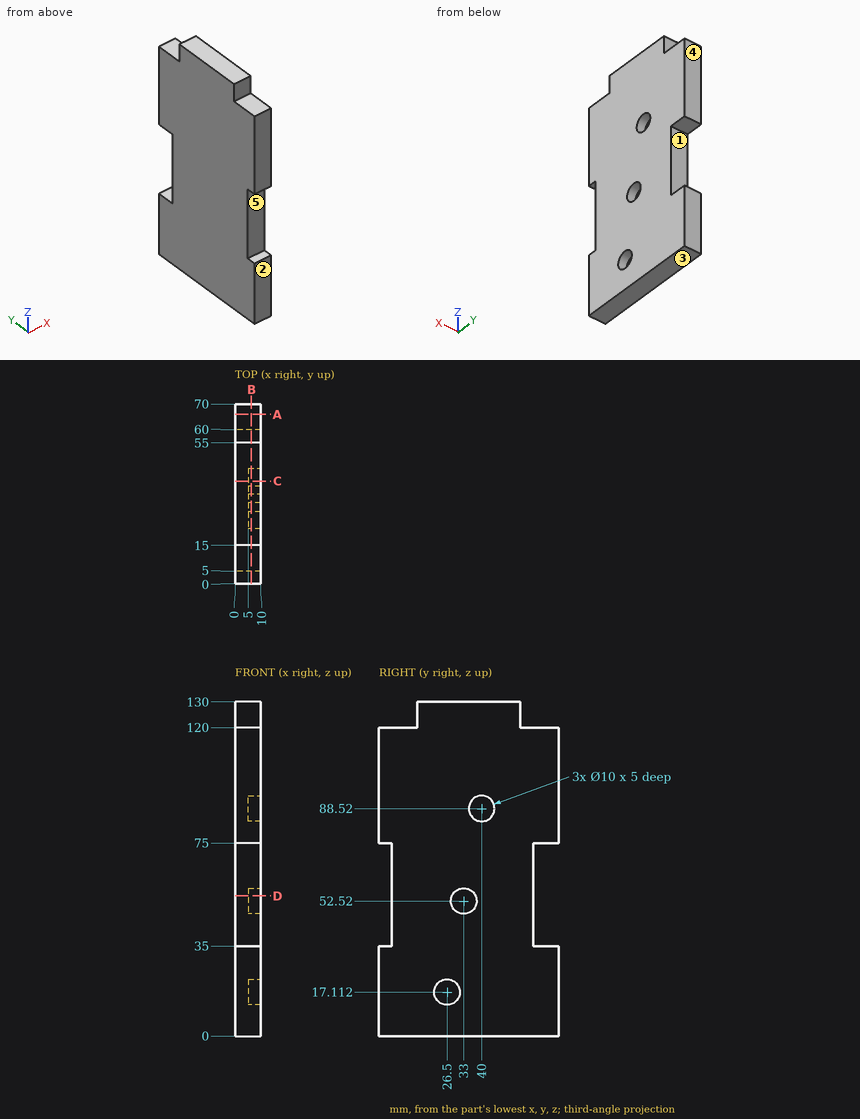
Job drawing, mm, ordinate dimensions from the low corner. One solid piece. A direction names the side the tool comes from. Give positions to 0.01 mm unless a question says otherwise; leave off trailing zeros. Loops run counter-clockwise (first coordinate to the right, second up) from the corner with the lowest first, then second, coordinate; pieces in that order, holes last. Notation, with made-up numbers: M 79,79 L 113,79 A31 ccw 113,110 Z; hole C 8.25,-39 d4. An arc over 180 degrees is marked long. Answer in a Markdown table with one row per item. Add a question column.
Item 1: Drop flat-ended pins along their axis: P1, Ø3, axis at x = 5, y = 63, coming from the +Z side; P2, Ø4, axis at y = 54.5, z = 26.5, coming from the -X side; P3, Ø5, axis at x = 4.5, z = 124.5, coming from the -Y side; P4, Ø5, axis at x = 6.5, z = 46.5, coming from the +Y side. Give the stop position or say it passes through.
Item 2: Tool access for the marked faces 1 and 2: list every direction of +Z, -Z, +X, -X, +Y, -Y with a clear straight run to the whole face (end or side of a thin tool).
Item 3: Band-saw the part on B-B on x = 6.25. Give the cut face in (y, z).
Item 4: Band-saw the part on D-D on z = 54.5. Give the cut face in (x, y).
Item 5: Band-saw the part on C-C on y = 40. Give the cut face in (x, z), then the cut area to 3 significant figures.
Item 6: Band-saw the part on A-A on y = 66. Give the cut face in (x, z), then the cut area to 3 significant figures.
Item 7: Mould opens along Z. For the marked faces 3, 4 and 5 say: +Z half, -Z half, draft (parallel to the pull), parting line (faces both ways), or undercut.
Item 8: Probe probe 1 along Z at (x, y) = (7.5, 62.5); probe 2 along Y at (x, z) = (7.65, 88.52); probe 3 along Y at (x, z) = (8.1, 52.52). List the from-to ranges inside material, lowest first.
Reply:
| question | item | result |
|---|---|---|
| 1 | P1 | stops at z = 120 |
| 1 | P2 | stops at x = 0 |
| 1 | P3 | stops at y = 15 |
| 1 | P4 | stops at y = 60 |
| 2 | face 1 | +X, -X, +Y |
| 2 | face 2 | +Z, -Z, +X, -X, -Y |
| 3 | outline | M 0,0 L 70,0 L 70,35 L 60,35 L 60,75 L 70,75 L 70,120 L 55,120 L 55,130 L 15,130 L 15,120 L 0,120 L 0,75 L 5,75 L 5,35 L 0,35 Z; hole C 26.5,17.11 d10; hole C 33,52.52 d10; hole C 40,88.52 d10 |
| 4 | outline | M 0,5 L 10,5 L 10,28.41 L 5,28.41 L 5,37.59 L 10,37.59 L 10,60 L 0,60 Z |
| 5 | outline | M 0,0 L 10,0 L 10,83.52 L 5,83.52 L 5,93.52 L 10,93.52 L 10,130 L 0,130 Z |
| 5 | area | 1,250 mm^2 |
| 6 | outline | M 0,0 L 10,0 L 10,35 L 0,35 Z; M 0,75 L 10,75 L 10,120 L 0,120 Z |
| 6 | area | 800 mm^2 |
| 7 | face 3 | -Z half |
| 7 | face 4 | draft |
| 7 | face 5 | undercut |
| 8 | probe 1 | z = 0 to 35, 75 to 120 |
| 8 | probe 2 | y = 0 to 35, 45 to 70 |
| 8 | probe 3 | y = 5 to 28, 38 to 60 |
